The model under review builds one solid part; all positions refer to its coordinate system, in mm. A direction names the side the tool comes from. Coordinates: 2 decimals unless noted, no trailing zeros. Order: outer loops, then holes, each group sorted by start corner. A loop starts at its lowest first (then second) coordinate and runs counter-clockwise, first axis right, second up. Notation, with made-up numbers: (-30, 62.25) -> (-26, 62.25) arc R3 cw to (-26, 66.25) -> close; hole circle Ø10 at (-33.5, 54). An arc over 180 degrees is marked (long way). Put each result on its own line as item: value.
from build123d import *

# Parameters (mm, degrees)
SKETCH3_R           = 50.2125
SKETCH3_R_2         = 49.2125
BOSS_EXTRUDE1_DEPTH = 702
SKETCH4_R           = 76
SKETCH4_R_2         = 49.2125
BOSS_EXTRUDE2_DEPTH = 1
SKETCH5_R           = 76
BOSS_EXTRUDE3_DEPTH = 1
BOSS_EXTRUDE4_DEPTH = 2
CIRPATTERN1_COUNT   = 4


with BuildPart() as part:
    # Sketch3 → Boss-Extrude1 (new body)
    with BuildSketch(Plane.XY):
        Circle(SKETCH3_R)
        Circle(SKETCH3_R_2, mode=Mode.SUBTRACT)
    extrude(amount=BOSS_EXTRUDE1_DEPTH)

    # Sketch4 → Boss-Extrude2 (add)
    with BuildSketch(Plane(origin=(0, 0, 0), x_dir=(-1, 0, 0), z_dir=(0, 0, -1))):
        Circle(SKETCH4_R)
        with Locations(Location((0, 0, 0), (0, 0, 180))):
            Circle(SKETCH4_R_2, mode=Mode.SUBTRACT)
    extrude(amount=-BOSS_EXTRUDE2_DEPTH)

    # Sketch5 → Boss-Extrude3 (add)
    with BuildSketch(Plane(origin=(0, 0, 100), x_dir=(-1, 0, 0), z_dir=(0, 0, -1))):
        Circle(SKETCH5_R)
    extrude(amount=-BOSS_EXTRUDE3_DEPTH)

    # Sketch6 → Boss-Extrude4 (add, symmetric)
    with BuildSketch(Plane(origin=(0, 0, 0), x_dir=(1, 0, 0), z_dir=(0, 1, 0))):
        Polygon((-49.2125, 0), (-49.2125, -350), (-249.2125, -100), (-249.2125, 0), align=None)
    boss_extrude4 = extrude(amount=BOSS_EXTRUDE4_DEPTH, both=True)

    # CirPattern1: Boss-Extrude4 ×4 about axis
    cirpattern1_axis = Axis((0, 0, 0), (0, 0, 1))
    for i in range(1, CIRPATTERN1_COUNT):
        add(boss_extrude4.rotate(cirpattern1_axis, i * 360 / CIRPATTERN1_COUNT))


solid = part.part
Item 1: Consider section C-C on y = -170.5. Write out the cut boundary in (x, z).
Answers below:
outline: (-2, 0) -> (2, 0) -> (2, 198.39) -> (-2, 198.39) -> close
Item 2: Mouldability with a two-part tool opening along Z and no side actions: class faces 1 (the flat face through (1, 1, 101)), 2 (the flat face through (40, 40, 1)), 3 (the cylindrical face through (-39.85, -30.55, 397.29)) as +Z half, -Z half, draft (parallel to the pull), parting line (faces both ways), or undercut.
Answers below:
face 1: +Z half
face 2: undercut
face 3: draft
Item 3: Consider section A-A on z = 84. Write out the cut boundary in (x, y) (1 decimal), and give its area (3 significant figures).
Answers below:
outline: (-249.2, -2) -> (-50.2, -2) arc R50.2 ccw to (-2, -50.2) -> (-2, -249.2) -> (2, -249.2) -> (2, -50.2) arc R50.2 ccw to (50.2, -2) -> (249.2, -2) -> (249.2, 2) -> (50.2, 2) arc R50.2 ccw to (2, 50.2) -> (2, 249.2) -> (-2, 249.2) -> (-2, 50.2) arc R50.2 ccw to (-50.2, 2) -> (-249.2, 2) -> close; hole circle Ø98.4 at (0, 0)
area: 3,500 mm^2
Item 4: Consider section D-D on x = 102.5. Write out the cut boundary in (y, z), and give its area (3 significant figures).
Answers below:
outline: (-2, 0) -> (2, 0) -> (2, 283.39) -> (-2, 283.39) -> close
area: 1,130 mm^2
Item 5: Consider section B-B on z = 271. Write out the cut boundary in (x, y) (1 decimal), and give its area (3 significant figures).
Answers below:
outline: (-112.4, -2) -> (-50.2, -2) arc R50.2 ccw to (-2, -50.2) -> (-2, -112.4) -> (2, -112.4) -> (2, -50.2) arc R50.2 ccw to (50.2, -2) -> (112.4, -2) -> (112.4, 2) -> (50.2, 2) arc R50.2 ccw to (2, 50.2) -> (2, 112.4) -> (-2, 112.4) -> (-2, 50.2) arc R50.2 ccw to (-50.2, 2) -> (-112.4, 2) -> close; hole circle Ø98.4 at (0, 0)
area: 1,310 mm^2
Item 6: For pin 1 Ø22 at (x, y) = (-32, 43) entering from +Z; pin 2 Ø1.5 at (x, z) = (-69, 230.5) entering from +Y, all flat-tipped, find the tip position at first contact; note any pin that passes through.
Answers below:
pin 1: z = 702
pin 2: y = 2
Item 7: For line 1 (Y direction, x = 0, z = 426); line 2 (Y direction, x = 0, z = 39); line 3 (Y direction, x = 138, z = 236), list the stretches that pass through material, from the lowest coordinate up. Write a range as from..to.
Answers below:
line 1: -50.21..-49.21, 49.21..50.21
line 2: -249.21..-49.21, 49.21..249.21
line 3: -2..2
Item 8: For faces 4 (the flat face through (-38, 40, 101)), 5 (the flat face through (40, 40, 101)), 6 (the cylindrical face through (-35.874, -35.133, 49.807)), 7 (the flat face through (-38, 40, 100)), 8 (the flat face through (40, -38, 100)), list the 3-axis set-ups (+Z, -Z, +X, -X, +Y, -Y) from which the entire face can be reached by the end or side of a thin tool; tool diameter is ignored.
Answers below:
face 4: +Z, -X, +Y
face 5: +Z, +X, +Y
face 6: -X, -Y
face 7: -X, +Y
face 8: +X, -Y
